Read the model definition and answer for the solid it produces. Units are mm, in the model's axes. Coordinates: 2 decimals unless noted, no trailing zeros. Loops run counter-clockwise (first coordinate to the right, second up) from the corner with the lowest first, then second, coordinate; pieces in that order, holes last. Notation, with made-up numbers: (-1.75, 28.5) - (13.25, 28.5) arc R17 ccw to (13.25, 54.5) - close; hole circle Ø6 at (50.25, 63). An arc over 180 degrees is marked (long way). Use CSV: the item, a comma, the result in double quotes.
```python
from build123d import *

# Parameters (mm, degrees)
F1_DEPTH = 76.2
F2_R     = 12.7
F3_SIZE  = 12.7


with BuildPart() as f1:
    # F0 (on Front) → F1 (new body)
    with BuildSketch(Plane.XZ):
        Polygon((35.114609, 27.737115), (-24.852807, 25.171665), (-15.263049, -29.26831), (37.456854, -27.012915), align=None)
    extrude(amount=F1_DEPTH)

    # F2
    f2_edges = [f1.edges().sort_by_distance(p)[0] for p in [
        (5.130901, -76.2, 26.45439),
        (36.285732, -76.2, 0.3621),
        (11.096903, -76.2, -28.140613),
        (-20.057928, -76.2, -2.048322),
    ]]
    fillet(f2_edges, radius=F2_R)

    # F3
    f3_edges = [f1.edges().sort_by_distance(p)[0] for p in [
        (11.096903, 0, -28.140613),
        (5.130901, 0, 26.45439),
        (36.285732, 0, 0.3621),
        (-20.057928, 0, -2.048322),
    ]]
    chamfer(f3_edges, length=F3_SIZE)


solid = f1.part
```
Q1. The part is cut by section A-A on y = -51.5. Determine the outline of the cut face in (x, z), and give its area (3 significant figures).
Reported:
outline,"(-24.85, 25.17) - (-15.26, -29.27) - (37.46, -27.01) - (35.11, 27.74) - close"
area,"3,090 mm²"
Q2. Find the intervals of material crossed by probe 1 along X at (y, z) = (-21, -16); probe 2 along X at (y, z) = (-38.5, 10.5); probe 3 along Y at (x, z) = (-9, -5.5), in increasing order. Write a range as [from, to].
Reported:
probe 1,"x = [-17.6, 36.99]"
probe 2,"x = [-22.27, 35.85]"
probe 3,"y = [-75.97, -2.41]"
Q3. Given P1, Ø8, axis at y = -62, z = -10, coming from the +X side; P2, Ø12, axis at x = 24, y = -63.5, coming from the +Z side; P3, Ø1.5, axis at x = 12.5, y = -27.5, coming from the +Z side, each flat-ended and moving along its own axis, determine where each tip first touches the part or whether it passes through.
Reported:
P1,"stops at x = 36.9"
P2,"stops at z = 27.52"
P3,"stops at z = 26.8"
Q4. The part is cut by section B-B on y = -64.5. Determine the outline of the cut face in (x, z).
Reported:
outline,"(-24.81, 25.13) - (-15.23, -29.23) - (37.42, -26.98) - (35.08, 27.7) - close"
